The model under review builds one solid part; all positions refer to its coordinate system, in mm. Face numbers are marked on the shaded views. A direction names the side the tool comes from. Round coordinates to 2 decimals unless told otherwise and drop trailing zeros. Loops run counter-clockwise (first coordinate to the right, second up) from the corner with the lowest first, then second, coordinate; pieces in that order, holes last. Notation, with made-up numbers: M 3,-27 L 26,-27 A8 cw 26,-17 Z; hole C -39.75,-8 d7. An arc over 180 degrees is marked long. Answer in a Markdown table with one row per item. Add a question column.
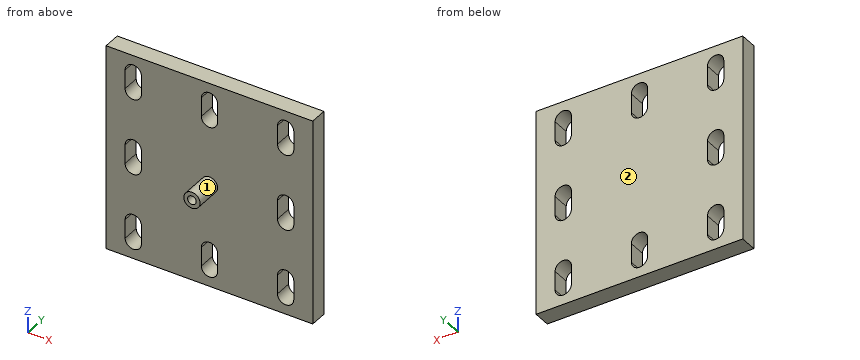
from build123d import *

# Parameters (mm, degrees)
SKETCH1_W           = 76.2
SKETCH1_H           = 76.2
BOSS_EXTRUDE1_DEPTH = 6.35
SKETCH2_R           = 3
BOSS_EXTRUDE2_DEPTH = 10
SKETCH3_R           = 1.5875
CUT_EXTRUDE1_DEPTH  = 10
CUT_EXTRUDE2_DEPTH  = 17.35


with BuildPart() as part:
    # Sketch1 → Boss-Extrude1 (new body)
    with BuildSketch(Plane(origin=(0, 0, 0), x_dir=(1, 0, 0), z_dir=(0, 1, 0))):
        Rectangle(SKETCH1_W, SKETCH1_H)
    extrude(amount=BOSS_EXTRUDE1_DEPTH)

    # Sketch2 → Boss-Extrude2 (add)
    with BuildSketch(Plane.XZ):
        Circle(SKETCH2_R)
    extrude(amount=BOSS_EXTRUDE2_DEPTH)

    # Sketch3 → Cut-Extrude1 (cut)
    with BuildSketch(Plane.XZ.offset(10)):
        Circle(SKETCH3_R)
    extrude(amount=-CUT_EXTRUDE1_DEPTH, mode=Mode.SUBTRACT)

    # Sketch5 → Cut-Extrude2 (cut, through all)
    with BuildSketch(Plane(origin=(0, 6.35, 0), x_dir=(1, 0, 0), z_dir=(0, 1, 0))):
        with BuildLine():
            Line((-25.1, 31.6), (-25.1, 24.6))
            ThreePointArc((-25.1, 24.6), (-28.1, 21.6), (-31.1, 24.6))
            Line((-31.1, 24.6), (-31.1, 31.6))
            ThreePointArc((-31.1, 31.6), (-28.1, 34.6), (-25.1, 31.6))
        make_face()
        with BuildLine():
            Line((-3, 31.6), (-3, 24.6))
            ThreePointArc((-3, 24.6), (0, 21.6), (3, 24.6))
            Line((3, 24.6), (3, 31.6))
            ThreePointArc((3, 31.6), (0, 34.6), (-3, 31.6))
        make_face()
        with BuildLine():
            Line((25.1, 31.6), (25.1, 24.6))
            ThreePointArc((25.1, 24.6), (28.1, 21.6), (31.1, 24.6))
            Line((31.1, 24.6), (31.1, 31.6))
            ThreePointArc((31.1, 31.6), (28.1, 34.6), (25.1, 31.6))
        make_face()
        with BuildLine():
            Line((25.1, 3.5), (25.1, -3.5))
            ThreePointArc((25.1, -3.5), (28.1, -6.5), (31.1, -3.5))
            Line((31.1, -3.5), (31.1, 3.5))
            ThreePointArc((31.1, 3.5), (28.1, 6.5), (25.1, 3.5))
        make_face()
        with BuildLine():
            Line((-3, -24.6), (-3, -31.6))
            ThreePointArc((-3, -31.6), (0, -34.6), (3, -31.6))
            Line((3, -31.6), (3, -24.6))
            ThreePointArc((3, -24.6), (0, -21.6), (-3, -24.6))
        make_face()
        with BuildLine():
            Line((25.1, -24.6), (25.1, -31.6))
            ThreePointArc((25.1, -31.6), (28.1, -34.6), (31.1, -31.6))
            Line((31.1, -31.6), (31.1, -24.6))
            ThreePointArc((31.1, -24.6), (28.1, -21.6), (25.1, -24.6))
        make_face()
        with BuildLine():
            Line((-31.1, 3.5), (-31.1, -3.5))
            ThreePointArc((-31.1, -3.5), (-28.1, -6.5), (-25.1, -3.5))
            Line((-25.1, -3.5), (-25.1, 3.5))
            ThreePointArc((-25.1, 3.5), (-28.1, 6.5), (-31.1, 3.5))
        make_face()
        with BuildLine():
            Line((-31.1, -24.6), (-31.1, -31.6))
            ThreePointArc((-31.1, -31.6), (-28.1, -34.6), (-25.1, -31.6))
            Line((-25.1, -31.6), (-25.1, -24.6))
            ThreePointArc((-25.1, -24.6), (-28.1, -21.6), (-31.1, -24.6))
        make_face()
    extrude(amount=-CUT_EXTRUDE2_DEPTH, mode=Mode.SUBTRACT)


solid = part.part
1. Take a section at C-C, the plane x = 0. State the section outline as (y, z) points, and give its area (3 significant figures).
2. Take a section at B-B, the plane z = 0. State the section outline as (x, y) points, and give its area (3 significant figures).
3. To check wall thickness, follow probe 1 along X at (y, z) = (0.75, 31); probe 2 along Z at (x, y) = (0, -2.5); probe 3 along X at (y, z) = (5.5, -24). State the ranges of each line that lie inside material, in increasing order.
4. Machinability: for the marked faces 1 and 2, which of the approach directions +Z, -Z, +X, -X, +Y, -Y give a long, thin tool a straight path to every point of the face, cutting with its end or side? Answer none if there is none.
5. Take a section at D-D, the plane y = -7.75. State the section outline as (x, z) points (1 decimal), and give its area (3 significant figures).
6. Take a section at A-A, the plane x = -28.1. State the section outline as (y, z) points.
7. For pin 1 Ø10 at (x, z) = (-0.5, 17.5) entering from -Y, flat-tipped, find the tip position at first contact; note if it passes through.
Check sheet entries:
| question | item | result |
|---|---|---|
| 1 | outline | M -10,-3 L 0,-3 L 0,-21.6 L 6.35,-21.6 L 6.35,21.6 L 0,21.6 L 0,3 L -10,3 L -10,1.59 L 0,1.59 L 0,-1.59 L -10,-1.59 Z; M 0,-38.1 L 6.35,-38.1 L 6.35,-34.6 L 0,-34.6 Z; M 0,34.6 L 6.35,34.6 L 6.35,38.1 L 0,38.1 Z |
| 1 | area | 347 mm^2 |
| 2 | outline | M -38.1,0 L -31.1,0 L -31.1,6.35 L -38.1,6.35 Z; M -25.1,0 L -3,0 L -3,-10 L -1.59,-10 L -1.59,0 L 1.59,0 L 1.59,-10 L 3,-10 L 3,0 L 25.1,0 L 25.1,6.35 L -25.1,6.35 Z; M 31.1,0 L 38.1,0 L 38.1,6.35 L 31.1,6.35 Z |
| 2 | area | 436 mm^2 |
| 3 | probe 1 | x = -38.1 to -31.1, -25.1 to -3, 3 to 25.1, 31.1 to 38.1 |
| 3 | probe 2 | z = -3 to -1.59, 1.59 to 3 |
| 3 | probe 3 | x = -38.1 to -31.04, -25.16 to -2.94, 2.94 to 25.16, 31.04 to 38.1 |
| 4 | face 1 | -Y |
| 4 | face 2 | +Z, -Z, +X, -X, +Y |
| 5 | outline | C 0,0 d6; hole C 0,0 d3.2 |
| 5 | area | 20.4 mm^2 |
| 6 | outline | M 0,-38.1 L 6.35,-38.1 L 6.35,-34.6 L 0,-34.6 Z; M 0,-21.6 L 6.35,-21.6 L 6.35,-6.5 L 0,-6.5 Z; M 0,6.5 L 6.35,6.5 L 6.35,21.6 L 0,21.6 Z; M 0,34.6 L 6.35,34.6 L 6.35,38.1 L 0,38.1 Z |
| 7 | pin 1 | stops at y = 0 |
